Check sheet for the modelled part. Datum: model origin and axes. Units: mm. Face numbers are marked on the shaded views. A direction names the side the tool comes from. Round coordinates to 2 decimals unless told otherwise and drop trailing zeros. Order: outer loops, then holes, each group sorted by start corner. A loop starts at its lowest first (then second) coordinate and runs counter-clockwise, first axis right, second up. Notation, with made-up numbers: (-17.75, -0.75) -> (-1.75, -0.75) arc R18 cw to (-1.75, 27.25) -> close; hole circle Ø11 at (20, 42.5). An arc over 180 degrees is marked (long way). Answer in a Markdown table with one row per item.
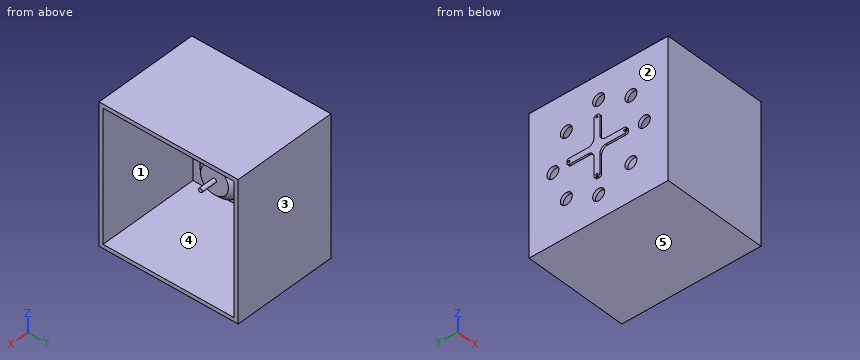
```python
from build123d import *

# Parameters (mm, degrees)
SKETCH1_R           = 12.7
BOSS_EXTRUDE1_DEPTH = 15.24
CHAMFER1_SIZE       = 3.81
CHAMFER3_SIZE       = 5.08
CHAMFER3_SIZE2      = 2.932939367
SKETCH2_R           = 1.27
BOSS_EXTRUDE3_DEPTH = 10.16
SKETCH3_R           = 0.639919682
SKETCH3_R_2         = 0.635
BOSS_EXTRUDE5_DEPTH = 1.27
SKETCH4_W           = 88.9
SKETCH4_H           = 88.9
BOSS_EXTRUDE6_DEPTH = 2.032
SKETCH5_R           = 3.81
CUT_EXTRUDE2_DEPTH  = 44.942
BOSS_EXTRUDE7_DEPTH = 1.27
SKETCH8_R           = 0.635
SKETCH8_R_2         = 0.639919682
CUT_EXTRUDE3_DEPTH  = 1.27
SKETCH9_W           = 88.9
SKETCH9_H           = 88.9
SKETCH9_W_2         = 83.82
SKETCH9_H_2         = 83.82
BOSS_EXTRUDE8_DEPTH = 80
SKETCH11_W          = 15.24
SKETCH11_H          = 88.9
CUT_EXTRUDE4_DEPTH  = 89.9


with BuildPart() as part:
    # Sketch1 → Boss-Extrude1 (new body, symmetric)
    with BuildSketch(Plane(origin=(0, 0, 0), x_dir=(0, 0, -1), z_dir=(1, 0, 0))):
        Circle(SKETCH1_R)
    extrude(amount=BOSS_EXTRUDE1_DEPTH, both=True)

    # Chamfer1
    chamfer1_edges = [part.edges().sort_by_distance(p)[0] for p in [
        (15.24, 0, 12.7),
    ]]
    chamfer(chamfer1_edges, length=CHAMFER1_SIZE)

    # Chamfer3
    chamfer3_edges = [part.edges().sort_by_distance(p)[0] for p in [
        (-15.24, 0, 12.7),
    ]]
    chamfer3_side = [part.faces().sort_by_distance(p)[0] for p in [
        (-15.24, 0, 0),
    ]]
    chamfer(chamfer3_edges, length=CHAMFER3_SIZE, length2=CHAMFER3_SIZE2, reference=chamfer3_side[0])

    # Sketch2 → Boss-Extrude3 (add)
    with BuildSketch(Plane(origin=(15.24, 0, 0), x_dir=(0, 0, -1), z_dir=(1, 0, 0))):
        Circle(SKETCH2_R)
    extrude(amount=BOSS_EXTRUDE3_DEPTH)

    # Sketch3 → Boss-Extrude5 (add)
    with BuildSketch(Plane.ZY.offset(15.24)):
        with BuildLine():
            Line((-5.715, -1.905), (-17.78, -1.905))
            ThreePointArc((-17.78, -1.905), (-18.678025612, -1.533025612), (-19.05, -0.635))
            Line((-19.05, -0.635), (-19.05, 0.635))
            ThreePointArc((-19.05, 0.635), (-18.678025612, 1.533025612), (-17.78, 1.905))
            Line((-17.78, 1.905), (-5.715, 1.905))
            ThreePointArc((-5.715, 1.905), (-3.020923164, 3.020923164), (-1.905, 5.715))
            Line((-1.905, 5.715), (-1.905, 17.78))
            ThreePointArc((-1.905, 17.78), (-1.533025612, 18.678025612), (-0.635, 19.05))
            Line((-0.635, 19.05), (0.635, 19.05))
            ThreePointArc((0.635, 19.05), (1.533025612, 18.678025612), (1.905, 17.78))
            Line((1.905, 17.78), (1.905, 5.715))
            ThreePointArc((1.905, 5.715), (3.020923164, 3.020923164), (5.715, 1.905))
            Line((5.715, 1.905), (17.78, 1.905))
            ThreePointArc((17.78, 1.905), (18.678025612, 1.533025612), (19.05, 0.635))
            Line((19.05, 0.635), (19.05, -0.635))
            ThreePointArc((19.05, -0.635), (18.678025612, -1.533025612), (17.78, -1.905))
            Line((17.78, -1.905), (5.715, -1.905))
            ThreePointArc((5.715, -1.905), (3.020923164, -3.020923164), (1.905, -5.715))
            Line((1.905, -5.715), (1.905, -17.78))
            ThreePointArc((1.905, -17.78), (1.533025612, -18.678025612), (0.635, -19.05))
            Line((0.635, -19.05), (-0.635, -19.05))
            ThreePointArc((-0.635, -19.05), (-1.533025612, -18.678025612), (-1.905, -17.78))
            Line((-1.905, -17.78), (-1.905, -5.715))
            ThreePointArc((-1.905, -5.715), (-3.020923164, -3.020923164), (-5.715, -1.905))
        make_face()
        with Locations((0, -17.78)):
            Circle(SKETCH3_R, mode=Mode.SUBTRACT)
        with Locations((17.78, 0)):
            Circle(SKETCH3_R_2, mode=Mode.SUBTRACT)
        with Locations((0, 17.78)):
            Circle(SKETCH3_R_2, mode=Mode.SUBTRACT)
        with Locations((-17.78, 0)):
            Circle(SKETCH3_R_2, mode=Mode.SUBTRACT)
    extrude(amount=BOSS_EXTRUDE5_DEPTH)

    # Sketch4 → Boss-Extrude6 (add)
    with BuildSketch(Plane.ZY.offset(16.51)):
        Rectangle(SKETCH4_W, SKETCH4_H)
    extrude(amount=BOSS_EXTRUDE6_DEPTH)

    # Sketch5 → Cut-Extrude2 (cut, through all)
    with BuildSketch(Plane.ZY.offset(18.542)):
        with Locations((0, 29.21)):
            Circle(SKETCH5_R)
        with Locations((20.654589078, 20.654589078)):
            Circle(SKETCH5_R)
        with Locations((29.21, 0)):
            Circle(SKETCH5_R)
        with Locations((20.654589078, -20.654589078)):
            Circle(SKETCH5_R)
        with Locations((0, -29.21)):
            Circle(SKETCH5_R)
        with Locations((-20.654589078, -20.654589078)):
            Circle(SKETCH5_R)
        with Locations((-29.21, 0)):
            Circle(SKETCH5_R)
        with Locations((-20.654589078, 20.654589078)):
            Circle(SKETCH5_R)
    extrude(amount=-CUT_EXTRUDE2_DEPTH, mode=Mode.SUBTRACT)

    # Sketch7 → Boss-Extrude7 (add)
    with BuildSketch(Plane.ZY.offset(18.542)):
        with BuildLine():
            Line((1.905, 5.715), (1.905, 7.378033275))
            Line((1.905, 7.378033275), (1.905, 17.78))
            ThreePointArc((1.905, 17.78), (1.533025612, 18.678025612), (0.635, 19.05))
            Line((0.635, 19.05), (-0.635, 19.05))
            ThreePointArc((-0.635, 19.05), (-1.533025612, 18.678025612), (-1.905, 17.78))
            Line((-1.905, 17.78), (-1.905, 5.715))
            ThreePointArc((-1.905, 5.715), (-3.020923164, 3.020923164), (-5.715, 1.905))
            Line((-5.715, 1.905), (-7.378033275, 1.905))
            Line((-7.378033275, 1.905), (-17.78, 1.905))
            ThreePointArc((-17.78, 1.905), (-18.678025612, 1.533025612), (-19.05, 0.635))
            Line((-19.05, 0.635), (-19.05, -0.635))
            ThreePointArc((-19.05, -0.635), (-18.678025612, -1.533025612), (-17.78, -1.905))
            Line((-17.78, -1.905), (-7.378033275, -1.905))
            Line((-7.378033275, -1.905), (-5.715, -1.905))
            ThreePointArc((-5.715, -1.905), (-3.020923164, -3.020923164), (-1.905, -5.715))
            Line((-1.905, -5.715), (-1.905, -7.378033275))
            Line((-1.905, -7.378033275), (-1.905, -17.78))
            ThreePointArc((-1.905, -17.78), (-1.533025612, -18.678025612), (-0.635, -19.05))
            Line((-0.635, -19.05), (0.635, -19.05))
            ThreePointArc((0.635, -19.05), (1.533025612, -18.678025612), (1.905, -17.78))
            Line((1.905, -17.78), (1.905, -7.378033275))
            Line((1.905, -7.378033275), (1.905, -5.715))
            ThreePointArc((1.905, -5.715), (3.020923164, -3.020923164), (5.715, -1.905))
            Line((5.715, -1.905), (7.378033275, -1.905))
            Line((7.378033275, -1.905), (17.78, -1.905))
            ThreePointArc((17.78, -1.905), (18.678025612, -1.533025612), (19.05, -0.635))
            Line((19.05, -0.635), (19.05, 0.635))
            ThreePointArc((19.05, 0.635), (18.678025612, 1.533025612), (17.78, 1.905))
            Line((17.78, 1.905), (7.378033275, 1.905))
            Line((7.378033275, 1.905), (5.715, 1.905))
            ThreePointArc((5.715, 1.905), (3.020923164, 3.020923164), (1.905, 5.715))
        make_face()
    extrude(amount=BOSS_EXTRUDE7_DEPTH)

    # Sketch8 → Cut-Extrude3 (cut)
    with BuildSketch(Plane.ZY.offset(19.812)):
        with Locations((0, 17.78)):
            Circle(SKETCH8_R)
        with Locations((17.78, 0)):
            Circle(SKETCH8_R)
        with Locations((0, -17.78)):
            Circle(SKETCH8_R_2)
        with Locations((-17.78, 0)):
            Circle(SKETCH8_R)
    extrude(amount=-CUT_EXTRUDE3_DEPTH, mode=Mode.SUBTRACT)

    # Sketch9 → Boss-Extrude8 (add)
    with BuildSketch(Plane(origin=(-16.51, 0, 0), x_dir=(0, 0, -1), z_dir=(1, 0, 0))):
        Rectangle(SKETCH9_W, SKETCH9_H)
        Rectangle(SKETCH9_W_2, SKETCH9_H_2, mode=Mode.SUBTRACT)
    extrude(amount=BOSS_EXTRUDE8_DEPTH)

    # Sketch11 → Cut-Extrude4 (cut, through all)
    with BuildSketch(Plane.XY.offset(44.45)):
        with Locations((55.87, 0)):
            Rectangle(SKETCH11_W, SKETCH11_H)
    extrude(amount=-CUT_EXTRUDE4_DEPTH, mode=Mode.SUBTRACT)


solid = part.part
```
(1) Section check B-B on y = -29.21. Record the boundary of the cut face in (x, z), plus the area to 3 significant figures.
Solutions:
| item | result |
|---|---|
| outline | (-18.54, -44.45) -> (48.25, -44.45) -> (48.25, -41.91) -> (-16.51, -41.91) -> (-16.51, -3.81) -> (-18.54, -3.81) -> close; (-18.54, 3.81) -> (-16.51, 3.81) -> (-16.51, 41.91) -> (48.25, 41.91) -> (48.25, 44.45) -> (-18.54, 44.45) -> close |
| area | 494 mm^2 |
(2) Draft check along Y on the marked faces 1, 2 and 3. Enter one of: pulls with the +Y half, pulls with the -Y half, needs draft (parallel to the pull), parting line crosses it, or undercut.
Solutions:
| item | result |
|---|---|
| face 1 | undercut |
| face 2 | needs draft |
| face 3 | pulls with the +Y half |
(3) Section check A-A on x = 22. Record the boundary of the cut face in (y, z).
Solutions:
| item | result |
|---|---|
| outline | (-44.45, -44.45) -> (44.45, -44.45) -> (44.45, 44.45) -> (-44.45, 44.45) -> close; circle Ø2.54 at (0, 0); hole (-41.91, -41.91) -> (41.91, -41.91) -> (41.91, 41.91) -> (-41.91, 41.91) -> close |
(4) Scan lines: probe 1 along Y at (x, z) = (-19, 0) (3 decimals); probe 2 along Z at (x, y) = (33, 34). Record each from-to range of solid material in increasing order. Write a range as from..to.
Solutions:
| item | result |
|---|---|
| probe 1 | -19.05..-18.42, -17.14..17.145, 18.415..19.05 |
| probe 2 | -44.45..-41.91, 41.91..44.45 |
(5) Section check D-D on x = 2.5. Record the boundary of the cut face in (y, z), plus the area to 3 significant figures.
Solutions:
| item | result |
|---|---|
| outline | (-44.45, -44.45) -> (44.45, -44.45) -> (44.45, 44.45) -> (-44.45, 44.45) -> close; circle Ø25.4 at (0, 0); hole (-41.91, -41.91) -> (41.91, -41.91) -> (41.91, 41.91) -> (-41.91, 41.91) -> close |
| area | 1,380 mm^2 |
(6) Depth check by flat-ended pin: pin 1 Ø0.6 at (x, y) = (-19, -0.5) entering from +Z; pin 2 Ø1.9 at (y, z) = (0.5, 11.5) entering from +X; pin 3 Ø7 at (y, z) = (-29.21, 0) entering from +X; pin 4 Ø2 at (y, z) = (26.5, 11.5) entering from -X. Enter the tip coordinate at first touch or a pass-through.
Solutions:
| item | result |
|---|---|
| pin 1 | z = 19.05 |
| pin 2 | x = 13.57 |
| pin 3 | through |
| pin 4 | x = -18.54 |
(7) Tool access check on the marked faces 4 and 5. Record the directions out of +Z, -Z, +X, -X, +Y, -Y that give a thin tool (end or side, any length) a straight path to the whole face; none if there is none.
Solutions:
| item | result |
|---|---|
| face 4 | +X |
| face 5 | -Z, +X, -X, +Y, -Y |
